CAD build for the part. Positions are in the model's coordinates, mm. A direction names the side the tool comes from. Round coordinates to 2 decimals unless told otherwise and drop trailing zeros. Order: outer loops, then holes, each group sorted by start corner. A loop starts at its lowest first (then second) coordinate and runs counter-clockwise, first axis right, second up. Notation, with made-up numbers: (7.5, 76.5) - (39.5, 76.5) arc R19 cw to (39.5, 101.5) - close; hole circle Ø2 at (-25.75, 58). An arc over 180 degrees is marked (long way). Write item = value, one per line.
Autodesk Inventor part; units mm, degrees
ref_plane "YZ Plane" through (0, 0, 0) normal (1, 0, 0) x (0, 1, 0)
ref_plane "XZ Plane" through (0, 0, 0) normal (0, 1, 0) x (-1, 0, 0)
ref_plane "XY Plane" through (0, 0, 0) normal (0, 0, 1) x (1, 0, 0)
sketch "Sketch1" plane through (0, 0, 0) normal (0, 0, 1) x (1, 0, 0)
  line L0 (-22.5075, -0.5954) -> (22.4925, -0.5954)
  line L1 (22.4925, -0.5954) -> (22.4925, 0.4046)
  line L2 (-22.5075, -0.5954) -> (-23.5075, -0.5954)
  line L3 (-23.5075, -0.5954) -> (-23.5075, 0.4046)
  line L4 (-22.5075, 2.4046) -> (22.4925, 2.4046)
  line L5 (22.4925, 2.4046) -> (22.4925, 0.4046)
  line L6 (22.4925, 0.4046) -> (23.4925, 0.4046)
  line L7 (23.4925, 0.4046) -> (23.4925, -0.5954)
  line L8 (23.4925, -0.5954) -> (22.4925, -0.5954)
  line L9 (-23.5075, 0.4046) -> (-22.5075, 0.4046)
  line L10 (-22.5075, 2.4046) -> (-22.5075, 0.4046)
  point P0 (0, 0)
  dimension "d2" = 1
  dimension "d3" = 1
  dimension "d5" = 1
  dimension "d6" = 1
  dimension "d7" = 3
  dimension "d11" = 2
extrude "Extrusion1" add sketch "Sketch1" along normal blind 60
fillet "Fillet1" radius 1 1 edges at (-0.0075, 2.4046, 60)
properties part number "upper coverr_3DPrint"
(1) Tool access for faces 1 (the flat face through (-22.508, 1, 30)), 2 (the flat face through (0, 1, 0)), 3 (the flat face through (22.492, 1, 30)): list every direction of +Z, -Z, +X, -X, +Y, -Y with a clear straight run to the whole face (end or side of a thin tool).
Solved:
face_1 = +Z, -Z, -X, +Y
face_2 = -Z, +X, -X, +Y, -Y
face_3 = +Z, -Z, +X, +Y
(2) Band-saw the part on A-A on z = 28. List the corners of the cut face in (x, y).
Solved:
outline = (-23.51, -0.6) - (23.49, -0.6) - (23.49, 0.4) - (22.49, 0.4) - (22.49, 2.4) - (-22.51, 2.4) - (-22.51, 0.4) - (-23.51, 0.4) - close
(3) Drop flat-ended pins along their axis: pin 1 (1 mm diameter, centred on y = 1, z = 14, fed in from -X); pin 2 (0.8 mm diameter, centred on x = -23.5, z = 32.5, fed in from +Y); pin 3 (1.6 mm diameter, centred on y = 1.5, z = 21, fed in from +X). Give the stop position or say it passes through.
Solved:
pin_1 = -22.51
pin_2 = 0.4
pin_3 = 22.49
(4) Probe line 1 along X through (y, z) = (1.35, 44.5); line 2 along Z through (x, y) = (-6, 1.7); line 3 along Z through (x, y) = (7, 1.95). List the from-to ranges inside material, lowest first.
Solved:
line_1 = -22.51 to 22.49
line_2 = 0 to 59.96
line_3 = 0 to 59.84
(5) Band-saw the part on B-B on y = 0.9. List the corners of the cut face in (x, z), plus the area to 3 significant figures.
Solved:
outline = (-22.51, 0) - (22.49, 0) - (22.49, 60) - (-22.51, 60) - close
area = 2,700 mm²
